Model file for the job. Use its own axes, mm. A direction names the side the tool comes from. Round coordinates to 2 decimals unless told otherwise and drop trailing zeros. Loops run counter-clockwise (first coordinate to the right, second up) from the corner with the lowest first, then second, coordinate; pieces in that order, holes last. Notation, with made-up numbers: M -0.75,5.5 L 10.25,5.5 A26 ccw 10.25,32.5 Z; hole C 34,64.5 d7. An arc over 180 degrees is marked long. Use a Markdown table: item, result. Add a question column.
Q1. Cut at B-B (x = -3). Give the cut face in (y, z).
Q2. Cut at D-D (z = -39). Give the cut face in (x, y).
Q3. Tool access for faces 1 (the face through (-3, -230, -28)), 2 (the face through (-3, -108, 0)), 3 (the face through (-2.71, -232.77, -55.51)): list every direction of +Z, -Z, +X, -X, +Y, -Y with a clear straight run to the whole face (end or side of a thin tool).
Q4. Cut at C-C (z = -55). Give the cut face in (x, y).
Q5. Mould opens along X. For faces 4 (the face through (-8.828, -146, 0)), 5 (the face through (-3, -226, -3)), 6 (the face through (-4.2, -232.7, -50.58)) say: +X half, -X half, draft (parallel to the pull), parting line (faces both ways), or undercut.
Q6. Cut at A-A (y = -235). Give the cut face in (x, z), plus the area to 3 significant figures.
Q7. Pin check, flat tips, straight feed: pin 1 (1.7 mm diameter, centred on y = 6, z = 1.5, fed in from -X); pin 2 (3 mm diameter, centred on x = -2.5, y = -104, fed in from -Z); pin 3 (3.5 mm diameter, centred on y = 4, z = 1, fed in from +X); pin 4 (3 mm diameter, centred on x = -7, z = -0.5, fed in from +Y). Stop position of each tip, or through.
Q8. Probe line 1 (Y direction, x = -5.8, z = 1.5); line 2 (Z direction, x = -5.5, y = -64); line 3 (Y direction, x = -5, z = -38.5). List the from-to ranges inside material, lowest first. Write a range as from..to.
from build123d import *

# Parameters (mm, degrees)
SKETCH2_W           = 6
SKETCH2_H           = 240
BOSS_EXTRUDE1_DEPTH = 3
BOSS_EXTRUDE2_DEPTH = 240
SKETCH5_W           = 3
SKETCH5_H           = 3
BOSS_EXTRUDE3_DEPTH = 10
SKETCH6_R           = 0.75
CUT_EXTRUDE1_DEPTH  = 40
SKETCH7_W           = 11.65685425
SKETCH7_H           = 10
BOSS_EXTRUDE4_DEPTH = 50.58
SKETCH8_R           = 2.25
BOSS_EXTRUDE5_DEPTH = 10
BOSS_EXTRUDE6_DEPTH = 11.656854


with BuildPart() as part:
    # Sketch2 → Boss-Extrude1 (new body)
    with BuildSketch(Plane.XY):
        with Locations((-3, -120)):
            Rectangle(SKETCH2_W, SKETCH2_H)
    extrude(amount=BOSS_EXTRUDE1_DEPTH)

    # Sketch4 → Boss-Extrude2 (add)
    with BuildSketch(Plane(origin=(0, -240, 0), x_dir=(-1, 0, 0), z_dir=(0, -1, 0))):
        Polygon((0, 0), (-2.828427125, 2.828427125), (-2.828427125, -3), (0, -3), align=None)
        Polygon((8.828427125, -3), (6, -3), (6, 0), (8.828427125, 2.828427125), align=None)
    extrude(amount=-BOSS_EXTRUDE2_DEPTH)

    # Sketch5 → Boss-Extrude3 (add)
    with BuildSketch(Plane(origin=(0, 0, 0), x_dir=(1, 0, 0), z_dir=(0, 1, 0))):
        with Locations((-6.5, -1.5)):
            Rectangle(SKETCH5_W, SKETCH5_H)
        with Locations((0.5, -1.5)):
            Rectangle(SKETCH5_W, SKETCH5_H)
    extrude(amount=BOSS_EXTRUDE3_DEPTH)

    # Sketch6 → Cut-Extrude1 (cut)
    with BuildSketch(Plane(origin=(2, 0, 0), x_dir=(0, 0, -1), z_dir=(1, 0, 0))):
        with Locations((-1.5, 6)):
            Circle(SKETCH6_R)
    extrude(amount=-CUT_EXTRUDE1_DEPTH, mode=Mode.SUBTRACT)

    # Sketch7 → Boss-Extrude4 (add)
    with BuildSketch(Plane(origin=(0, 0, 0), x_dir=(-1, 0, 0), z_dir=(0, 0, -1))):
        with Locations((3, -235)):
            Rectangle(SKETCH7_W, SKETCH7_H)
    extrude(amount=BOSS_EXTRUDE4_DEPTH)

    # Sketch8 → Boss-Extrude5 (add)
    with BuildSketch(Plane(origin=(0, 0, -50.58), x_dir=(-1, 0, 0), z_dir=(0, 0, -1))):
        with Locations((3, -235)):
            Circle(SKETCH8_R)
    extrude(amount=BOSS_EXTRUDE5_DEPTH)

    # Sketch9 → Boss-Extrude6 (add)
    with BuildSketch(Plane.ZY.offset(8.828427125)):
        Polygon((-7, -230), (0, -230), (0, -223), align=None)
    extrude(amount=-BOSS_EXTRUDE6_DEPTH)


solid = part.part
Checked values:
| question | item | result |
|---|---|---|
| 1 | outline | M -240,-50.58 L -237.25,-50.58 L -237.25,-60.58 L -232.75,-60.58 L -232.75,-50.58 L -230,-50.58 L -230,-7 L -223,0 L 0,0 L 0,3 L -240,3 Z |
| 2 | outline | M -8.83,-240 L 2.83,-240 L 2.83,-230 L -8.83,-230 Z |
| 3 | face 1 | -Z, +X, -X, +Y |
| 3 | face 2 | -Z, +Y |
| 3 | face 3 | -Z |
| 4 | outline | C -3,-235 d4.5 |
| 5 | face 4 | -X half |
| 5 | face 5 | undercut |
| 5 | face 6 | draft |
| 6 | outline | M -8.83,-50.58 L -5.25,-50.58 L -5.25,-60.58 L -0.75,-60.58 L -0.75,-50.58 L 2.83,-50.58 L 2.83,3 L -8.83,3 Z |
| 6 | area | 670 mm^2 |
| 7 | pin 1 | stops at x = -8 |
| 7 | pin 2 | stops at z = 0 |
| 7 | pin 3 | stops at x = 2 |
| 7 | pin 4 | stops at y = 10 |
| 8 | line 1 | y = -240..5.25, 6.75..10 |
| 8 | line 2 | z = 0..3 |
| 8 | line 3 | y = -240..-230 |
